The listing builds one solid part. Answer for the finished solid, in the listing's coordinates (mm). Face numbers are marked on the shaded views. A direction names the side the tool comes from. Coordinates: 2 decimals unless noted, no trailing zeros. Order: outer loops, then holes, each group sorted by start corner. A loop starts at its lowest first (then second) coordinate and runs counter-clockwise, first axis right, second up. Notation, with made-up numbers: (-36, 76) -> (-24, 76) arc R18 ccw to (-24, 105) -> close; hole circle Ø3 at (36, -19). An arc over 180 degrees is marked (long way). One line per question, with ' | ' between items.
from build123d import *

# Parameters (mm, degrees)
F0_W     = 23
F0_H     = 3
F1_DEPTH = 2
F2_DEPTH = 6


with BuildPart() as f1:
    # F0 (on Top) → F1 (new body)
    with BuildSketch(Plane.XY):
        with BuildLine():
            Line((-11, -7.5), (11, -7.5))
            ThreePointArc((11, -7.5), (18.5, 0), (11, 7.5))
            Line((11, 7.5), (-11, 7.5))
            ThreePointArc((-11, 7.5), (-18.5, 0), (-11, -7.5))
        make_face()
        with Locations((0, -4)):
            Rectangle(F0_W, F0_H, mode=Mode.SUBTRACT)
        with Locations((0, 4)):
            Rectangle(F0_W, F0_H, mode=Mode.SUBTRACT)
        with BuildLine():
            Line((11, 17.5), (-11, 17.5))
            ThreePointArc((-11, 17.5), (-28.5, 0), (-11, -17.5))
            Line((-11, -17.5), (11, -17.5))
            ThreePointArc((11, -17.5), (28.5, 0), (11, 17.5))
        make_face()
        with BuildLine():
            ThreePointArc((11, 7.5), (18.5, 0), (11, -7.5))
            Line((11, -7.5), (-11, -7.5))
            ThreePointArc((-11, -7.5), (-18.5, 0), (-11, 7.5))
            Line((-11, 7.5), (11, 7.5))
        make_face(mode=Mode.SUBTRACT)
    extrude(amount=F1_DEPTH)

    # F0 (on Top) → F2 (join)
    with BuildSketch(Plane.XY):
        with BuildLine():
            Line((-11, -7.5), (11, -7.5))
            ThreePointArc((11, -7.5), (18.5, 0), (11, 7.5))
            Line((11, 7.5), (-11, 7.5))
            ThreePointArc((-11, 7.5), (-18.5, 0), (-11, -7.5))
        make_face()
        with Locations((0, -4)):
            Rectangle(F0_W, F0_H, mode=Mode.SUBTRACT)
        with Locations((0, 4)):
            Rectangle(F0_W, F0_H, mode=Mode.SUBTRACT)
    extrude(amount=F2_DEPTH)


solid = f1.part
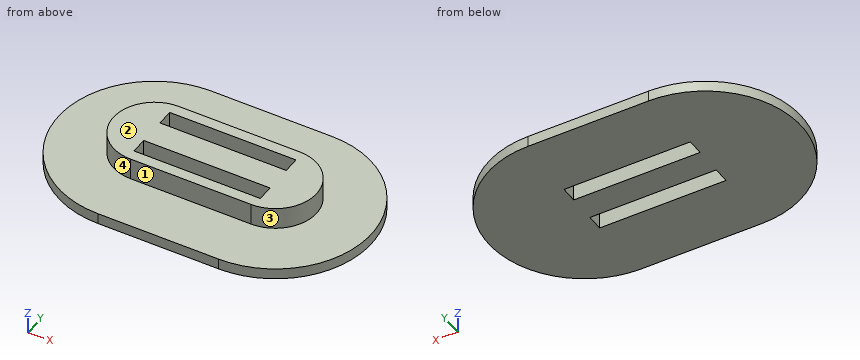
Item 1: Find the intervals of material crossed by L1, parallel to Y at x = 0, z = 3.7; L2, parallel to Y at x = 7, z = 1.8; L3, parallel to Z at x = 18, y = 8, in increasing order.
Computed values:
L1: y = -7.5 to -5.5, -2.5 to 2.5, 5.5 to 7.5 | L2: y = -17.5 to -5.5, -2.5 to 2.5, 5.5 to 17.5 | L3: z = 0 to 2
Item 2: Section C-C, the plane y = 0 is taken. Give the vertices of the cut face in (x, z), plus the area to 3 significant figures.
Computed values:
outline: (-28.5, 0) -> (28.5, 0) -> (28.5, 2) -> (18.5, 2) -> (18.5, 6) -> (-18.5, 6) -> (-18.5, 2) -> (-28.5, 2) -> close | area: 262 mm^2
Item 3: Section B-B, the plane y = 4 is taken. Give the vertices of the cut face in (x, z).
Computed values:
outline: (-28.04, 0) -> (-11.5, 0) -> (-11.5, 6) -> (-17.34, 6) -> (-17.34, 2) -> (-28.04, 2) -> close; (11.5, 0) -> (28.04, 0) -> (28.04, 2) -> (17.34, 2) -> (17.34, 6) -> (11.5, 6) -> close
Item 4: Section D-D, the plane x = -15 is taken. Give the vertices of the cut face in (y, z), plus the area to 3 significant figures.
Computed values:
outline: (-17.04, 0) -> (17.04, 0) -> (17.04, 2) -> (6.34, 2) -> (6.34, 6) -> (-6.34, 6) -> (-6.34, 2) -> (-17.04, 2) -> close | area: 119 mm^2
Item 5: Section A-A, the plane z = 0.95 is taken. Give the vertices of the cut face in (x, y).
Computed values:
outline: (-11, -17.5) -> (11, -17.5) arc R17.5 ccw to (11, 17.5) -> (-11, 17.5) arc R17.5 ccw to start; hole (-11.5, -5.5) -> (11.5, -5.5) -> (11.5, -2.5) -> (-11.5, -2.5) -> close; hole (-11.5, 2.5) -> (11.5, 2.5) -> (11.5, 5.5) -> (-11.5, 5.5) -> close
Item 6: For the marked faces 1, 2, 3 and 4, determine the directions among +Z, -Z, +X, -X, +Y, -Y from which every point of the face is accessible in a straight line to the end or side of a thin tool.
Computed values:
face 1: +Z, +X, -X, -Y | face 2: +Z, +X, -X, +Y, -Y | face 3: +Z, +X | face 4: +Z, -X
Item 7: Each of these flat-tipped pins is pushed along its axis until it touches: pin 1 Ø4 at (x, y) = (-19.5, -3.5) entering from +Z; pin 2 Ø3 at (x, z) = (16.5, 3) entering from -Y; pin 3 Ø1.5 at (y, z) = (-4.5, 4) entering from +X; pin 4 Ø0.9 at (y, z) = (4, 2) entering from +X. Where does it stop, or does it pass through?
Computed values:
pin 1: stops at z = 6 | pin 2: stops at y = -16.94 | pin 3: stops at x = 17.5 | pin 4: stops at x = 28.14
